from build123d import *

# Parameters (mm, degrees)
ESQUISSE1_W             = 70
ESQUISSE1_H             = 41
BOSS_EXTRU_1_DEPTH      = 3
COQUE1_T                = -2.2
CHANFREIN1_SIZE         = 2
ESQUISSE3_W             = 20.2
ESQUISSE3_H             = 15.2
ENL_V_MAT_EXTRU_2_DEPTH = 1.6
ENL_V_MAT_EXTRU_5_DEPTH = 41.672472263
ENL_V_START             = -2.2
ENL_V_MAT_EXTRU_4_DEPTH = 2.2
ESQUISSE7_W             = 65.6
ESQUISSE7_H             = 36.6
ESQUISSE7_W_2           = 61.6
ESQUISSE7_H_2           = 32.6
EXTRU_MINCE1_DEPTH      = 2
CONG_1_R                = 1


# Read off the part's stored shape, not the designer's step: Enlèv. mat.-Extru.4
with BuildPart() as part:
    # Esquisse1 → Boss.-Extru.1 (new body)
    with BuildSketch(Plane(origin=(0, 0, 0), x_dir=(1, 0, 0), z_dir=(0, 1, 0))):
        Rectangle(ESQUISSE1_W, ESQUISSE1_H)
    extrude(amount=BOSS_EXTRU_1_DEPTH)

    # Coque1
    coque1_openings = [part.faces().sort_by_distance(p)[0] for p in [
        (0, 0, 0),
    ]]
    offset(amount=COQUE1_T, openings=coque1_openings, kind=Kind.INTERSECTION)

    # Chanfrein1
    chanfrein1_edges = [part.edges().sort_by_distance(p)[0] for p in [
        (-35, 3, 0),
        (0, 3, 20.5),
        (35, 3, 0),
        (35, 1.5, 20.5),
        (-35, 1.5, 20.5),
        (-35, 1.5, -20.5),
        (35, 1.5, -20.5),
        (0, 3, -20.5),
    ]]
    chamfer(chanfrein1_edges, length=CHANFREIN1_SIZE)

    # Esquisse3 → Enlèv. mat.-Extru.2 (cut)
    with BuildSketch(Plane.XZ.offset(-0.8)):
        with Locations((-17, 0)):
            Rectangle(ESQUISSE3_W, ESQUISSE3_H)
    extrude(amount=-ENL_V_MAT_EXTRU_2_DEPTH, mode=Mode.SUBTRACT)

    # Esquisse8 → Enlèv. mat.-Extru.5 (cut, through all)
    with BuildSketch(Plane(origin=(0, 3, 0), x_dir=(1, 0, 0), z_dir=(0, 1, 0))):
        with BuildLine():
            Line((-13.9, 5.056854249), (-13.9, 0.6))
            ThreePointArc((-13.9, 0.6), (-14.5, 0), (-15.1, 0.6))
            Line((-15.1, 0.6), (-15.1, 5.056854249))
            ThreePointArc((-15.1, 5.056854249), (-14.5, 5.656854249), (-13.9, 5.056854249))
        make_face()
        with BuildLine():
            ThreePointArc((-17.752691193, 3.252691193), (-14.5, -4.6), (-11.247308807, 3.252691193))
            ThreePointArc((-11.247308807, 3.252691193), (-12.095836944, 3.252691193), (-12.095836944, 2.404163056))
            ThreePointArc((-12.095836944, 2.404163056), (-14.5, -3.4), (-16.904163056, 2.404163056))
            ThreePointArc((-16.904163056, 2.404163056), (-16.904163056, 3.252691193), (-17.752691193, 3.252691193))
        make_face()
    extrude(amount=-ENL_V_MAT_EXTRU_5_DEPTH, mode=Mode.SUBTRACT)

    # Enlèv. mat.-Extru.4 outline → Enlèv. mat.-Extru.4 (cut)
    with BuildSketch(Plane(origin=(0, 3, 0), x_dir=(1, 0, 0), z_dir=(0, 1, 0)).offset(ENL_V_START)):
        Polygon((21.667594623, 5.714552033), (24.142355296, 7.1431654), (14.244110438, 12.858801818), (14.243939692, 10.001279345), align=None)
        Polygon((12.5925129, -0.475203574), (5.9935572, 3.335122269), (5.993101889, -4.284757181), (12.592057589, -8.095083023), align=None)
        Polygon((4.344642768, 4.288171287), (1.870052841, 5.717080393), (1.869369857, -5.7130095), (4.34413053, -4.284396133), align=None)
        Polygon((12.594164363, 10.001377924), (12.594335108, 12.858900397), (2.695407267, 7.144446922), (5.169997194, 5.715537816), align=None)
        Polygon((5.168559477, -5.714552033), (2.693798804, -7.1431654), (12.592043662, -12.858801818), (12.592214408, -10.001279345), align=None)
        Polygon((14.240438301, -8.095181519), (20.839849312, -4.28564432), (20.840304623, 3.33423513), (14.240893612, -0.47530207), align=None)
        Polygon((13.418138159, 0.954049774), (20.01754917, 4.763586973), (13.41859347, 8.573912816), (6.819182459, 4.764375617), align=None)
        Polygon((22.491511493, -4.285480495), (24.96610142, -5.714389602), (24.966784403, 5.715700292), (22.49202373, 4.287086925), align=None)
        Polygon((14.241989737, -10.001377924), (14.241818992, -12.858900397), (24.140746833, -7.144446922), (21.666156906, -5.715537816), align=None)
    extrude(amount=ENL_V_MAT_EXTRU_4_DEPTH, mode=Mode.SUBTRACT)

    # Esquisse7 → Extru.-Mince1 (add)
    with BuildSketch(Plane.XZ.offset(-0.8)):
        Rectangle(ESQUISSE7_W, ESQUISSE7_H)
        Rectangle(ESQUISSE7_W_2, ESQUISSE7_H_2, mode=Mode.SUBTRACT)
    extrude(amount=EXTRU_MINCE1_DEPTH)

    # Congé1
    cong_1_edges = [part.edges().sort_by_distance(p)[0] for p in [
        (-32.8, -0.6, -18.3),
        (32.8, -0.6, -18.3),
        (32.8, -0.6, 18.3),
        (-32.8, -0.6, 18.3),
        (0, 0.8, -16.3),
        (30.8, 0.8, 0),
        (0, 0.8, 16.3),
        (-30.8, 0.8, 0),
    ]]
    fillet(cong_1_edges, radius=CONG_1_R)


solid = part.part
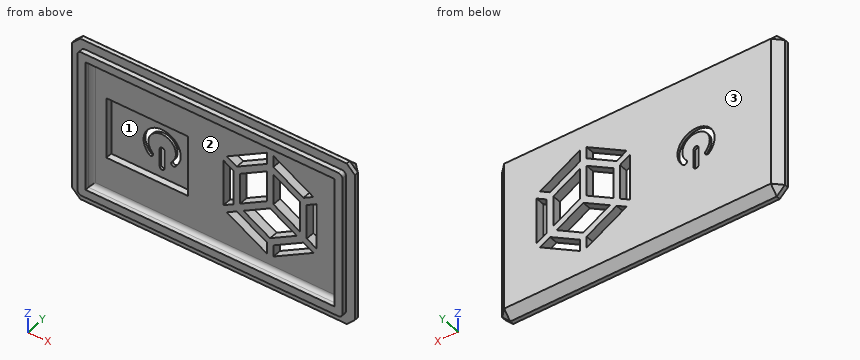
Input: part model. Units: mm. Frame: model coordinates. Face numbers are marked on the shaded views. Round coordinates to 2 decimals unless told otherwise and drop trailing zeros. Write each loop counter-clockwise with the first axis right and the second up, starting at its lowest first coordinate (ties: lowest second). Pieces come first, ordered by that corner, then holes.
1) Cut plane B-B (z = 12). Return the cut outline in (x, y).
2) Ray query, L1, parallel to Z at x = -14.5, y = 2.7; L2, parallel to Z at x = 12.5, y = 2.15; L3, parallel to Z at x = -14.5, y = 2.8. Return the intervals inside material, ascending.
3) Contact query for flat-ended pins moving along their axis: P1, Ø24.5, axis at x = -6.5, z = 1, coming from the -Y side; P2, Ø0.8, axis at y = -0.5, z = -3, coming from the -X side; P3, Ø1.3, axis at x = -18.5, y = 2, coming from the +Z side; P4, Ø2.5, axis at y = 1.5, z = -11, coming from the -X side. Output: stop coordinate, or through.
4) Cut plane A-A (x = 8.5). Count the separate pieces of the cut face and the enclosed holes in it, then the cut area to 3 significant figures.
5) Cut plane C-C (x = -8.5). Return the cut outline in (y, z), then the cut area to 3 significant figures.
6) Draft query along Z for the marked faces 1, 2 and 3. Return one class per face: pulls with the +Z half, pulls with the -Z half, needs draft (parallel to the pull), parting line crosses it, or undercut.
Geometry says:
1. outline: (-35, 0) - (-32.8, 0) - (-32.8, -1.2) - (-30.8, -1.2) - (-30.8, -0.2) arc R1 cw to (-29.8, 0.8) - (11.1, 0.8) - (11.1, 3) - (-33, 3) - (-35, 1) - close; (12.59, 0.8) - (14.24, 0.8) - (14.24, 3) - (12.59, 3) - close; (15.73, 0.8) - (29.8, 0.8) arc R1 cw to (30.8, -0.2) - (30.8, -1.2) - (32.8, -1.2) - (32.8, 0) - (35, 0) - (35, 1) - (33, 3) - (15.73, 3) - close
2. L1: z = -18.8 to -5.66, 0 to 3.4, 4.6 to 18.8
2. L2: z = -19.35 to -12.8, -9.95 to -8.04, -1.48 to 0.42, 8.04 to 9.95, 12.81 to 19.35
2. L3: z = -18.7 to -5.66, 0 to 3.4, 4.6 to 18.7
3. P1: stops at y = 0.8
3. P2: stops at x = -32.8
3. P3: stops at z = 20.15
3. P4: stops at x = -35
4. separate pieces: 5
4. enclosed holes: 0
4. area: 64.5 mm2
5. outline: (-1.2, -18.3) - (0, -18.3) - (0, -20.5) - (1, -20.5) - (3, -18.5) - (3, 18.5) - (1, 20.5) - (0, 20.5) - (0, 18.3) - (-1.2, 18.3) - (-1.2, 16.3) - (-0.2, 16.3) arc R1 cw to (0.8, 15.3) - (0.8, 7.6) - (2.4, 7.6) - (2.4, -7.6) - (0.8, -7.6) - (0.8, -15.3) arc R1 cw to (-0.2, -16.3) - (-1.2, -16.3) - close
5. area: 73.8 mm2
6. face 1: undercut
6. face 2: undercut
6. face 3: needs draft
